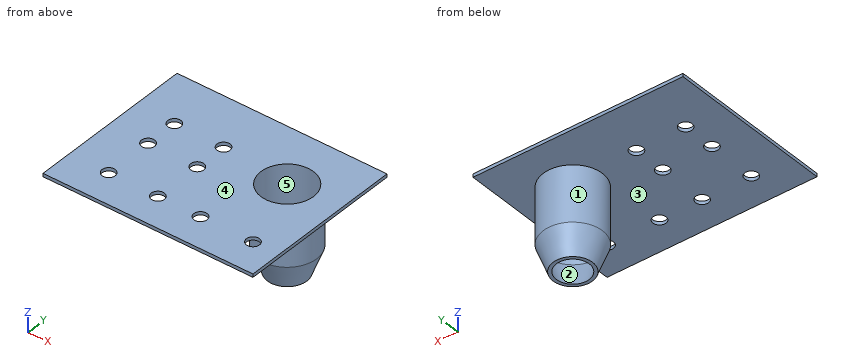
Autodesk Inventor part; units mm, degrees
ref_plane "YZ Plane" through (0, 0, 0) normal (1, 0, 0) x (0, 1, 0)
ref_plane "XZ Plane" through (0, 0, 0) normal (0, 1, 0) x (-1, 0, 0)
ref_plane "XY Plane" through (0, 0, 0) normal (0, 0, 1) x (1, 0, 0)
sketch "Sketch1" plane through (0, 0, 0) normal (0, 0, 1) x (1, 0, 0)
  line L0 (-48, 18) -> (16, 18)
  line L1 (16, 18) -> (16, -33)
  line L2 (16, -33) -> (-48, -33)
  line L3 (-48, -33) -> (-48, 18)
  circle A0 centre (0, 0) radius 8
  dimension "d0" = 64
  dimension "d1" = 51
  dimension "d2" = 18
  dimension "d3" = 16
  dimension "d4" = 16
extrude "Extrusion1" add sketch "Sketch1" along normal blind 1
sketch "Sketch2" plane through (0, 0, 1) normal (0, 0, 1) x (1, 0, 0)
  line L0 (-48, 18) -> (-48, -33)
  line L1 (-48, -33) -> (16, -33)
  point P0 (0, 0)
  point P1 (-36, 2)
  point P2 (-36, -8)
  point P3 (-36, -23)
  point P4 (-21, 2)
  point P5 (-21, -8)
  point P6 (-21, -23)
  point P7 (-8, -23)
  point P8 (8, -23)
  dimension "d7" = 12
  dimension "d8" = 15
  dimension "d9" = 13
  dimension "d10" = 16
  dimension "d11" = 10
  dimension "d12" = 15
  dimension "d13" = 10
hole "Hole1" at (-36, 2, 1) at (-36, -8, 1) at (-36, -23, 1) at (-21, 2, 1) at (-21, -8, 1) at (-21, -23, 1) at (-8, -23, 1) at (8, -23, 1) direction (0, 0, -1) diameter 4 end through all
sketch "Sketch7" plane through (0, 0, 0) normal (1, 0, 0) x (0, 1, 0)
  line L0 (8, 0) -> (-8, 0)
  line L1 (5, -25) -> (6, -25)
  line L2 (18, 0) -> (-33, 0)
  line L3 (8, 0) -> (9, 0)
  line L4 (0, -31.2) -> (0, 5.2)
  line L5 (9, 0) -> (9, -17)
  line L6 (9, -17) -> (6, -25)
  line L7 (8, 0) -> (8, -17)
  line L8 (8, -17) -> (5, -25)
  point P0 (0, 0)
  dimension "d33" = 25
  dimension "d34" = 1
  dimension "d35" = 5
  dimension "d37" = 17
revolve "Revolution1" add sketch "Sketch7" angle 360 about axis through (0, 0, -10) along (0, 0, 1)
sketch "Sketch8" plane through (0, 0, -25) normal (0, 0, -1) x (-1, 0, 0)
  point P0 (0, 0)
properties part number "OpeningV2"
Can you work these out from the model? Positions are in its coordinate system, mm. Face numbers are marked on the shaded views. A direction names the side the tool comes from. Round coordinates to 2 decimals unless told otherwise and drop trailing zeros. Loops run counter-clockwise (first coordinate to the right, second up) from the corner with the lowest first, then second, coordinate; pieces in that order, holes last. Notation, with made-up numbers: M 13,10.5 L 50,10.5 A26 ccw 50,45.5 Z; hole C 83.5,72 d7. An arc over 180 degrees is marked long. Answer as a JSON object with one key per item and string values. Group by question number.
Q1. Imagine slicing it at C-C, the plane y = -15. Please give me the cut outline in (x, z).
Q2. Please list where these lines run through material, in increasing order: L1, parallel to X at y = -23, z = 0.4; L2, parallel to Y at x = -36, z = 0.35; L3, parallel to X at y = 2, z = 0.65.
Q3. We'd pull the mould along X, two halves only. Please class the marked faces 1, 2 and 3: +X half, -X half, draft (parallel to the pull), parting line (faces both ways), or undercut.
Q4. Imagine slicing it at A-A, the plane x = -36. Please give me the cut outline in (y, z).
Q5. Imagine slicing it at D-D, the plane x = -28. Please give me the cut outline in (y, z), then the cut area to 3 significant figures.
Q6. Imagine slicing it at B-B, the plane z = -5. Please give me the cut outline in (x, y), then the cut area to 3 significant figures.
Q7. On a 3-axis mill with a long thin cutter (end or side, diameter ignored), from which of +Z, -Z, +X, -X, +Y, -Y can I reach the whole of each face in a straight line? I mean the marked faces 4 and 5. Say none if no direction works.
Q8. Will these pins go through, and if not, where does the flat tip stop? pin 1 (4.5 mm diameter, centred on x = 8, y = -23, fed in from -Z); pin 2 (3 mm diameter, centred on x = -8, y = -23, fed in from +Z); pin 3 (5 mm diameter, centred on x = -36, y = -23, fed in from +Z); pin 4 (3 mm diameter, centred on y = 0.5, z = -17.5, fed in from +X).
Findings:
{
 "1": {"outline": "M -48,0 L 16,0 L 16,1 L -48,1 Z"},
 "2": {"L1": "x = -48 to -38, -34 to -23, -19 to -10, -6 to 6, 10 to 16", "L2": "y = -33 to -25, -21 to -10, -6 to 0, 4 to 18", "L3": "x = -48 to -38, -34 to -23, -19 to -7.75, 7.75 to 16"},
 "3": {"face 1": "parting line", "face 2": "undercut", "face 3": "draft"},
 "4": {"outline": "M -33,0 L -25,0 L -25,1 L -33,1 Z; M -21,0 L -10,0 L -10,1 L -21,1 Z; M -6,0 L 0,0 L 0,1 L -6,1 Z; M 4,0 L 18,0 L 18,1 L 4,1 Z"},
 "5": {"outline": "M -33,0 L 18,0 L 18,1 L -33,1 Z", "area": "51.0 mm2"},
 "6": {"outline": "C 0,0 d18; hole C 0,0 d16", "area": "53.4 mm2"},
 "7": {"face 4": "+Z, +X, -X, +Y, -Y", "face 5": "+Z"},
 "8": {"pin 1": "stops at z = 0", "pin 2": "passes through", "pin 3": "stops at z = 1", "pin 4": "stops at x = 9"}
}
